Part model, mm, in its own coordinate system. Face numbers are marked on the shaded views. Give positions to 0.01 mm unless a question says otherwise; leave off trailing zeros. Write each loop counter-clockwise with the first axis right and the second up, starting at its lowest first coordinate (ties: lowest second). Pieces come first, ordered by that corner, then holes. Notation, with made-up numbers: (31.5, -19) - (80.5, -19) arc R32 ccw to (80.5, 20) - close; hole circle Ø4 at (52, 85). An arc over 180 degrees is marked (long way). Answer in a Markdown table with one row per item. Add a question column.
1. Probe line 1 along Y through (x, z) = (-7.25, -7); line 2 along X through (y, z) = (3.75, 0); line 3 along X through (y, z) = (2.35, -11). List the from-to ranges inside material, lowest first.
2. Band-saw the part on D-D on y = 0.35. Write the cut outline in (x, z).
3. Band-saw the part on A-A on y = 3.45. State how many separate pieces and enclosed holes the cut face has, plus the area to 3 significant figures.
4. Band-saw the part on C-C on x = 10.5. Write the cut outline in (y, z).
5. Band-saw the part on B-B on z = -10. Write the cut outline in (x, y).
6. Pull direction Z, two halves, no side cores. Call the marked faces 1, 2 and 3: released by +Z, released by -Z, zero draft, split by the parting line, or undercut.
7. Drop a flat-ended pin along its axis: pin 1 Ø1.5 at (x, y) = (-4, 2) entering from +Z. Give the stop position or say it passes through.
```python
from build123d import *

# Parameters (mm, degrees)
SKETCH_1_R          = 14.25
EXTRUDE_1_DEPTH     = 4
SKETCH_2_R          = 11.25
CUT_EXTRUDE_1_DEPTH = 1
EXTRUDE_2_DEPTH     = 1


with BuildPart() as part:
    # 草图1 → 凸台-拉伸1 (new body)
    with BuildSketch(Plane(origin=(0, 0, 0), x_dir=(1, 0, 0), z_dir=(0, 1, 0))):
        with Locations(Location((0, 0, 0), (0, 0, 270))):
            Circle(SKETCH_1_R)
    extrude(amount=EXTRUDE_1_DEPTH)

    # 草图2 → 切除-拉伸1 (cut)
    with BuildSketch(Plane(origin=(0, 4, 0), x_dir=(1, 0, 0), z_dir=(0, 1, 0))):
        with Locations(Location((0, 0, 0), (0, 0, 270))):
            Circle(SKETCH_2_R)
    extrude(amount=-CUT_EXTRUDE_1_DEPTH, mode=Mode.SUBTRACT)

    # 草图3 → 凸台-拉伸2 (add)
    with BuildSketch(Plane(origin=(0, 3, 0), x_dir=(1, 0, 0), z_dir=(0, 1, 0))):
        with BuildLine():
            ThreePointArc((-4, -2), (0, -6), (4, -2))
            add(Edge.make_bspline(
                [(4, -2), (4, 1.17143168), (1.660537063, 1.196977672), (0, 7)],
                knots=[0, 0, 0, 0, 1, 1, 1, 1], degree=3))
            add(Edge.make_bspline(
                [(-4, -2), (-4, 1.17143168), (-1.660537063, 1.196977672), (0, 7)],
                knots=[0, 0, 0, 0, 1, 1, 1, 1], degree=3))
        make_face()
    extrude(amount=EXTRUDE_2_DEPTH)


solid = part.part
```
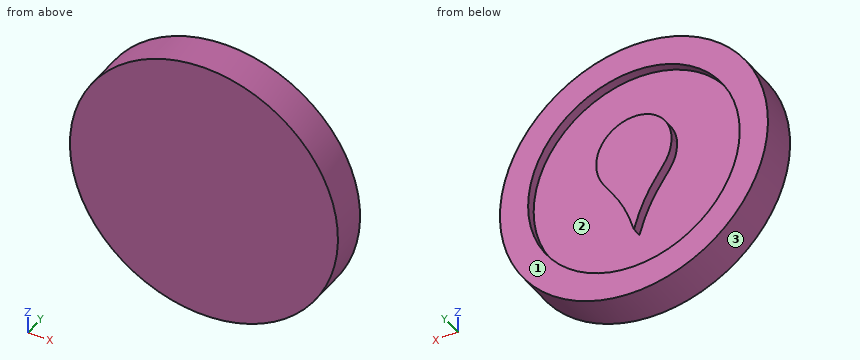
Values:
| question | item | result |
|---|---|---|
| 1 | line 1 | y = 0 to 3 |
| 1 | line 2 | x = -14.25 to -11.25, -3.58 to 3.58, 11.25 to 14.25 |
| 1 | line 3 | x = -9.06 to 9.06 |
| 2 | outline | circle Ø28.5 at (0, 0) |
| 3 | separate pieces | 2 |
| 3 | enclosed holes | 1 |
| 3 | area | 303 mm² |
| 4 | outline | (0, -9.63) - (4, -9.63) - (4, -4.04) - (3, -4.04) - (3, 4.04) - (4, 4.04) - (4, 9.63) - (0, 9.63) - close |
| 5 | outline | (-10.15, 0) - (10.15, 0) - (10.15, 4) - (5.15, 4) - (5.15, 3) - (-5.15, 3) - (-5.15, 4) - (-10.15, 4) - close |
| 6 | face 1 | zero draft |
| 6 | face 2 | undercut |
| 6 | face 3 | split by the parting line |
| 7 | pin 1 | stops at z = 13.87 |
